```python
from build123d import *

# Parameters (mm, degrees)
SKETCH_R        = 1.75
PAD_DEPTH       = 8.4
FILLET_R        = 2
CHAMFER001_SIZE = 2
CHAMFER_SIZE    = 0.5


with BuildPart() as part:
    # Sketch → Pad (new body)
    with BuildSketch(Plane.XY):
        with BuildLine():
            Line((-10, -5), (-5, -10))
            Line((-5, -10), (5, -10))
            Line((5, -10), (15, 0))
            Line((15, 0), (26.25, 0))
            ThreePointArc((33.75, 0), (30, 3.75), (26.25, 0))
            Line((33.75, 0), (45, 0))
            Line((45, 0), (55, -10))
            Line((55, -10), (65, -10))
            Line((65, -10), (70, -5))
            Line((70, -5), (70, 5))
            Line((70, 5), (50, 25))
            Line((50, 25), (10, 25))
            Line((10, 25), (-10, 5))
            Line((-10, 5), (-10, -5))
        make_face()
        Circle(SKETCH_R, mode=Mode.SUBTRACT)
        with Locations((15, 15)):
            Circle(SKETCH_R, mode=Mode.SUBTRACT)
        with Locations((45, 15)):
            Circle(SKETCH_R, mode=Mode.SUBTRACT)
        with Locations((60, 0)):
            Circle(SKETCH_R, mode=Mode.SUBTRACT)
    extrude(amount=PAD_DEPTH)

    # Fillet
    fillet_edges = [part.edges().sort_by_distance(p)[0] for p in [
        (33.75, 0, 4.2),
        (26.25, 0, 4.2),
    ]]
    fillet(fillet_edges, radius=FILLET_R)

    # Chamfer001
    chamfer001_edges = [part.edges().sort_by_distance(p)[0] for p in [
        (10, -5, 8.4),
        (50, -5, 8.4),
    ]]
    chamfer(chamfer001_edges, length=CHAMFER001_SIZE)

    # Chamfer
    chamfer_edges = [part.edges().sort_by_distance(p)[0] for p in [
        (40.195482, 0, 0),
        (34.248884, 0.358156, 0),
        (50, -5, 0),
        (30, 3.75, 0),
        (60, -10, 0),
        (25.751116, 0.358156, 0),
        (67.5, -7.5, 0),
        (19.804518, 0, 0),
        (70, 0, 0),
        (10, -5, 0),
        (60, 15, 0),
        (0, -10, 0),
        (30, 25, 0),
        (-7.5, -7.5, 0),
        (0, 15, 0),
        (-10, 0, 0),
        (58.25, 0, 0),
        (43.25, 15, 0),
        (13.25, 15, 0),
        (-1.75, 0, 0),
        (19.804518, 0, 8.4),
        (-1.414214, -10, 8.4),
        (61.414214, -10, 8.4),
        (67.5, -7.5, 8.4),
        (70, 0, 8.4),
        (-7.5, -7.5, 8.4),
        (-10, 0, 8.4),
        (0, 15, 8.4),
        (30, 25, 8.4),
        (60, 15, 8.4),
    ]]
    chamfer(chamfer_edges, length=CHAMFER_SIZE)


solid = part.part
```
Design review of the part built by this model. Coordinates are the model's own, in mm. A direction names the side the tool comes from. Round coordinates to 2 decimals unless told otherwise and drop trailing zeros. Write each loop counter-clockwise with the first axis right and the second up, starting at its lowest first coordinate (ties: lowest second). Pieces come first, ordered by that corner, then holes. Notation, with made-up numbers: (-5, -8) -> (19, -8) arc R8 ccw to (19, 0) -> close; hole circle Ø1 at (9, 30). An arc over 180 degrees is marked (long way). Answer in a Markdown table with one row per item.
Q1. Take a section at B-B, the plane y = 15. State the section outline as (x, z) points, then the cut area to 3 significant figures.
The answers:
| item | result |
|---|---|
| outline | (0, 0.5) -> (0.71, 0) -> (12.75, 0) -> (13.25, 0.5) -> (13.25, 8.4) -> (0.71, 8.4) -> (0, 7.9) -> close; (16.75, 0.5) -> (17.25, 0) -> (42.75, 0) -> (43.25, 0.5) -> (43.25, 8.4) -> (16.75, 8.4) -> close; (46.75, 0.5) -> (47.25, 0) -> (59.29, 0) -> (60, 0.5) -> (60, 7.9) -> (59.29, 8.4) -> (46.75, 8.4) -> close |
| area | 444 mm² |
Q2. Take a section at D-D, the plane y = 9. State the section outline as (x, z) points.
The answers:
| item | result |
|---|---|
| outline | (-6, 0.5) -> (-5.29, 0) -> (65.29, 0) -> (66, 0.5) -> (66, 7.9) -> (65.29, 8.4) -> (-5.29, 8.4) -> (-6, 7.9) -> close |
Q3. Take a section at A-A, the plane x = 0. State the section outline as (y, z) points.
The answers:
| item | result |
|---|---|
| outline | (-10, 0.5) -> (-9.5, 0) -> (-2.25, 0) -> (-1.75, 0.5) -> (-1.75, 8.4) -> (-9.5, 8.4) -> (-10, 7.9) -> close; (1.75, 0.5) -> (2.25, 0) -> (14.29, 0) -> (15, 0.5) -> (15, 7.9) -> (14.29, 8.4) -> (1.75, 8.4) -> close |
Q4. Draft analysis for pull direction X (two halves, no side actions). For faces 6 (the face through (20, 0, 4)), 7 (the face through (-10, 0, 4)), 8 (the face through (59.966, 14.686, 0.253)), state which applies: +X half, -X half, draft (parallel to the pull), parting line (faces both ways), or undercut.
The answers:
| item | result |
|---|---|
| face 6 | undercut |
| face 7 | -X half |
| face 8 | +X half |
Q5. For faces 1 (the face through (9.83, -4.82, 0.25)), 2 (the face through (10, -5, 3)), 3 (the face through (-7.36, -7.29, 8.15)), 4 (the face through (8.68, -4.89, 7.41)), 5 (the face through (46.669, 15.526, 4.395)), list the 3-axis set-ups (+Z, -Z, +X, -X, +Y, -Y) from which the entire face can be reached by the end or side of a thin tool; tool diameter is ignored.
The answers:
| item | result |
|---|---|
| face 1 | -Z, -Y |
| face 2 | +Z, -Z, -Y |
| face 3 | +Z, -X, -Y |
| face 4 | +Z, -Y |
| face 5 | +Z, -Z |
Q6. Clearance check with flat-ended pins moving along their axes: pin 1 Ø3 at (x, y) = (0, 0) entering from +Z; pin 2 Ø5 at (x, z) = (26, 6) entering from -Y; pin 3 Ø5 at (y, z) = (20.5, 2) entering from -X. State where each tip first meets the part, or that it passes through.
The answers:
| item | result |
|---|---|
| pin 1 | through |
| pin 2 | y = 0 |
| pin 3 | x = 3 |
Q7. Take a section at C-C, the plane z = 5.5. State the section outline as (x, y) points, then the cut area to 3 significant figures.
The answers:
| item | result |
|---|---|
| outline | (-10, -5) -> (-5, -10) -> (5, -10) -> (15, 0) -> (24.61, 0) arc R2 ccw to (26.48, 1.3) arc R3.75 cw to (33.52, 1.3) arc R2 ccw to (35.39, 0) -> (45, 0) -> (55, -10) -> (65, -10) -> (70, -5) -> (70, 5) -> (50, 25) -> (10, 25) -> (-10, 5) -> close; hole circle Ø3.5 at (0, 0); hole circle Ø3.5 at (15, 15); hole circle Ø3.5 at (45, 15); hole circle Ø3.5 at (60, 0) |
| area | 1,910 mm² |
Q8. To check wall thickness, follow L1, parallel to Y at x = 15, z = 6.5; L2, parallel to Y at x = 60, z = 5; L3, parallel to Y at x = 37, z = 4.5. State the ranges of each line that lie inside material, in increasing order. Write a range as [from, to].
The answers:
| item | result |
|---|---|
| L1 | [0, 13.25], [16.75, 25] |
| L2 | [-10, -1.75], [1.75, 15] |
| L3 | [0, 25] |
